```python
from build123d import *

# Parameters (mm, degrees)
F1_DEPTH = 6
F2_DEPTH = 2
F3_DEPTH = 25


with BuildPart() as f1:
    # F0 (on Top) → F1 (new body)
    with BuildSketch(Plane.XY):
        with BuildLine():
            Line((1.5, 30.9636884108), (1.5, 33.9668956486))
            ThreePointArc((1.5, 33.9668956486), (0, 34), (-1.5, 33.9668956486))
            Line((-1.5, 33.9668956486), (-1.5, 30.9636884108))
            ThreePointArc((-1.5, 30.9636884108), (0, 31), (1.5, 30.9636884108))
        make_face()
        with BuildLine():
            ThreePointArc((-1.5, 33.9668956486), (-23.5053185471, -24.5662369931), (34, 0))
            ThreePointArc((34, 0), (24.5662369931, 23.5053185471), (1.5, 33.9668956486))
            Line((1.5, 33.9668956486), (1.5, 30.9636884108))
            ThreePointArc((1.5, 30.9636884108), (22.4443756875, 21.3834047803), (31, 0))
            ThreePointArc((31, 0), (-21.3834047803, -22.4443756875), (-1.5, 30.9636884108))
            Line((-1.5, 30.9636884108), (-1.5, 33.9668956486))
        make_face()
    extrude(amount=F1_DEPTH)

    # F0 (on Top) → F2 (join)
    with BuildSketch(Plane.XY):
        with BuildLine():
            Line((1.5, 25.6097931415), (1.5, 30.9636884108))
            ThreePointArc((1.5, 30.9636884108), (0, 31), (-1.5, 30.9636884108))
            Line((-1.5, 30.9636884108), (-1.5, 25.6097931415))
            Line((-1.5, 25.6097931415), (1.5, 25.6097931415))
        make_face()
        with BuildLine():
            ThreePointArc((31, 0), (22.4443756875, 21.3834047803), (1.5, 30.9636884108))
            Line((1.5, 30.9636884108), (1.5, 25.6097931415))
            Line((1.5, 25.6097931415), (-1.5, 25.6097931415))
            Line((-1.5, 25.6097931415), (-1.5, 30.9636884108))
            ThreePointArc((-1.5, 30.9636884108), (-21.3834047803, -22.4443756875), (31, 0))
        make_face()
    extrude(amount=F2_DEPTH)

    # F0 (on Top) → F3 (cut)
    with BuildSketch(Plane.XY):
        with BuildLine():
            Line((1.5, 30.9636884108), (1.5, 33.9668956486))
            ThreePointArc((1.5, 33.9668956486), (0, 34), (-1.5, 33.9668956486))
            Line((-1.5, 33.9668956486), (-1.5, 30.9636884108))
            ThreePointArc((-1.5, 30.9636884108), (0, 31), (1.5, 30.9636884108))
        make_face()
    extrude(amount=F3_DEPTH, mode=Mode.SUBTRACT)


solid = f1.part
```
Part model, mm, in its own coordinate system. A direction names the side the tool comes from. Give positions to 0.01 mm unless a question says otherwise; leave off trailing zeros. Order: outer loops, then holes, each group sorted by start corner. A loop starts at its lowest first (then second) coordinate and runs counter-clockwise, first axis right, second up. Notation, with made-up numbers: M 14.25,43 L 26.25,43 A30 cw 26.25,73 Z; hole C -7,44 d10. An arc over 180 degrees is marked long. Use a Markdown table: item, result. Add a question column.
(1) Probe line 1 along X through (y, z) = (0, 3.5); line 2 along Z through (x, y) = (0, -22); line 3 along Y through (x, z) = (5, 5.6). List the from-to ranges inside material, lowest first. Write a range as [from, to].
(2) 3-axis set-ups, long thin cutter, end or side, ignore diameter. For faces 1 (the face through (-1.5, 32, 3)), 2 (the face through (0, 0, 0)): which of +Z, -Z, +X, -X, +Y, -Y reach the whole face in a straight line?
(3) Mould opens along Y. For faces 3 (the face through (0, 0, 2)), 4 (the face through (-1.47, -33.97, 2.96)), 5 (the face through (1.5, 32, 3)) say: +Y half, -Y half, draft (parallel to the pull), parting line (faces both ways), or undercut.
(4) Drop flat-ended pins along their axis: P1, Ø1.5, axis at x = 2.5, z = 2, coming from the -Y side; P2, Ø1.5, axis at x = -8, y = -15.5, coming from the +Z side; P3, Ø3.5, axis at y = 33, z = 3.5, coming from the -X side. Give the stop position or say it passes through.
(5) Saw through at A-A, the plane z = 4.6. Give the cut face in (x, y), and give its area (3 significant figures).
(6) Saw through at C-C, the plane x = -15. Give the cut face in (y, z).
(7) Saw through at B-B, the plane y = -28.5. Give the cut face in (x, z).
(8) Saw through at D-D, the plane x = 0. Give the cut face in (y, z).
Answer key:
| question | item | result |
|---|---|---|
| 1 | line 1 | [-34, -31], [31, 34] |
| 1 | line 2 | [0, 2] |
| 1 | line 3 | [-33.63, -30.59], [30.59, 33.63] |
| 2 | face 1 | +Z, -Z, +Y |
| 2 | face 2 | -Z, +X, -X, +Y, -Y |
| 3 | face 3 | undercut |
| 3 | face 4 | parting line |
| 3 | face 5 | draft |
| 4 | P1 | y = -33.95 |
| 4 | P2 | z = 2 |
| 4 | P3 | x = -13.4 |
| 5 | outline | M -1.5,30.96 L -1.5,33.97 A34 ccw long 1.5,33.97 L 1.5,30.96 A31 cw long Z |
| 5 | area | 604 mm^2 |
| 6 | outline | M -30.51,0 L 30.51,0 L 30.51,6 L 27.13,6 L 27.13,2 L -27.13,2 L -27.13,6 L -30.51,6 Z |
| 7 | outline | M -18.54,0 L 18.54,0 L 18.54,6 L 12.2,6 L 12.2,2 L -12.2,2 L -12.2,6 L -18.54,6 Z |
| 8 | outline | M -34,0 L 31,0 L 31,2 L -31,2 L -31,6 L -34,6 Z |
